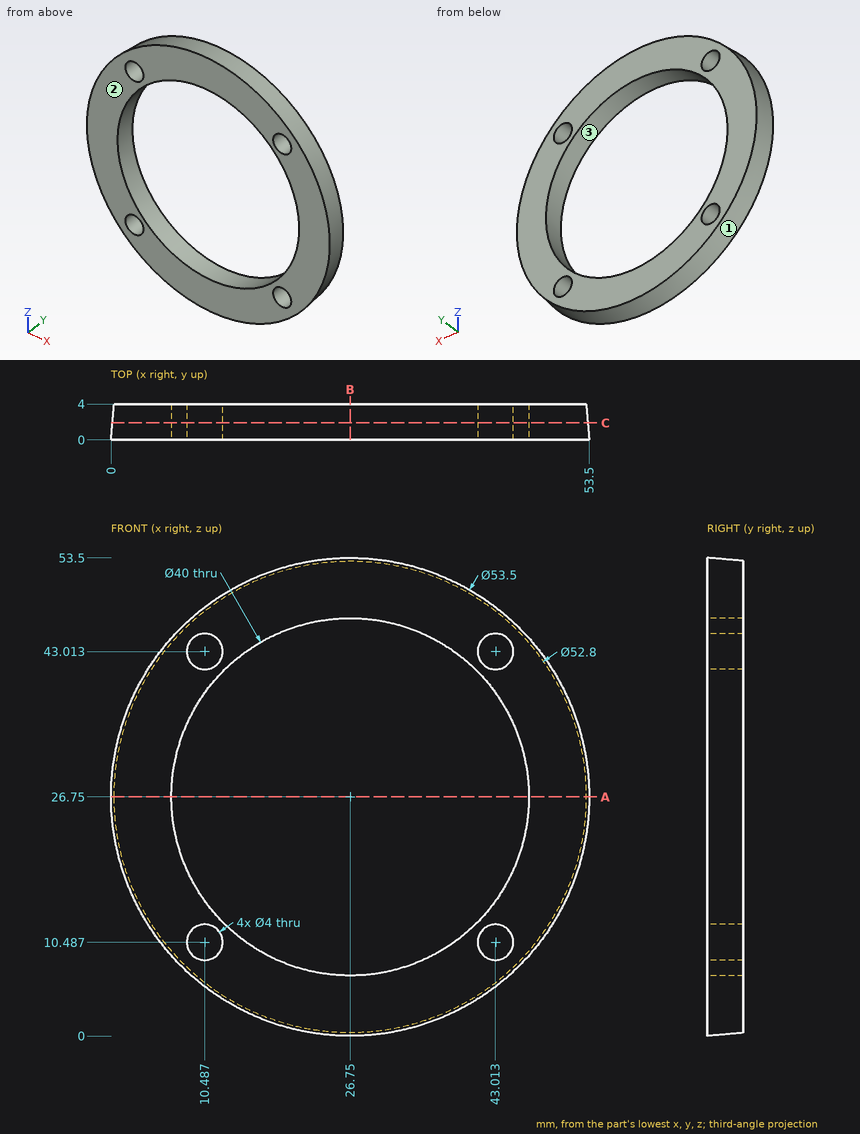
Check sheet for the drawn part. Datum: minimum x, y, z corner. Units: mm. Coordinates: 2 decimals unless noted, no trailing zeros. Order: outer loops, then holes, each group sorted by start corner. A loop starts at its lowest first (then second) coordinate and runs counter-clockwise, first axis right, second up. Notation, with made-up numbers: M 45,6 L 57,6 A26 ccw 57,25 Z; hole C 86,15.25 d9. An arc over 180 degrees is marked long. One line per question, with ' | ' between items. Start each with the question number.
Item 1: Cross-section at A-A on z = 26.75. Enter the section's corners in (x, y), then the cut area to 3 significant figures.
Item 2: Draft check along X on the marked faces 1, 2 and 3. Enter one of: pulls with the +X half, pulls with the -X half, needs draft (parallel to the pull), parting line crosses it, or undercut.
Item 3: Cross-section at B-B on x = 26.75. Enter the section's corners in (y, z).
Item 4: Cross-section at C-C on y = 1.9. Enter the section's corners in (x, z).
Item 5: Material ranges on L1, parallel to Z at x = 18, y = 0.35 (1 decimal); L2, parallel to X at y = 1.5, z = 15 (1 decimal); L3, parallel to X at y = 1.9, z = 28.5, recorded low to high. Write a range as [from, to].
Item 6: Gauge pin test, flat end, axial feed: pin 1 (1.5 mm diameter, centred on y = 2, z = 41, fed in from +X). Record the tip position at first contact, or that the pin passes through.
Findings:
1) outline: M 0,0 L 6.75,0 L 6.75,4 L 0.35,4 Z; M 46.75,0 L 53.5,0 L 53.15,4 L 46.75,4 Z | area: 52.6 mm²
2) face 1: parting line crosses it | face 2: needs draft | face 3: undercut
3) outline: M 0,0 L 4,0.35 L 4,6.75 L 0,6.75 Z; M 0,46.75 L 4,46.75 L 4,53.15 L 0,53.5 Z
4) outline: C 26.75,26.75 d53.17; hole C 26.75,26.75 d40; hole C 10.49,10.49 d4; hole C 10.49,43.01 d4; hole C 43.01,10.49 d4; hole C 43.01,43.01 d4
5) L1: z = [1.5, 8.8], [44.7, 52] | L2: x = [2.9, 10.6], [42.9, 50.6] | L3: x = [0.22, 6.83], [46.67, 53.28]
6) pin 1: stops at x = 49.65
